Source: CAD feature listing. Evaluate the final solid. Frame: model axes, mm. Face numbers are marked on the shaded views. A direction names the side the tool comes from. Give positions to 0.01 mm unless a question says otherwise; leave off trailing zeros. Order: outer loops, then holes, each group sorted by start corner. A loop starts at its lowest first (then second) coordinate and runs counter-clockwise, first axis right, second up.
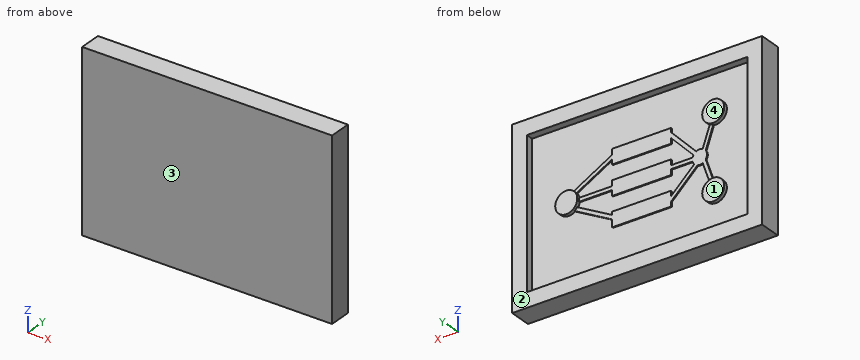
from build123d import *

# Parameters (mm, degrees)
CROQUIS1_W              = 34
CROQUIS1_H              = 24
SALIENTE_EXTRUIR1_DEPTH = 3
CAVIDAD1_START          = 2
CAVIDAD1_OUTLINE_W      = 30
CAVIDAD1_OUTLINE_H      = 20
CAVIDAD1_DEPTH          = 1
CAVIDAD1_START_2        = 2.15
CAVIDAD1_2_DEPTH        = 0.85
CAVIDAD1_START_3        = 2.5
CAVIDAD1_3_OUTLINE_R    = 1.5
CAVIDAD1_3_DEPTH        = 0.5
SALIENTE_EXTRUIR3_DEPTH = 0.5
CROQUIS6_W              = 7.77529117
CROQUIS6_H              = 2
CROQUIS6_W_2            = 2
CROQUIS6_H_2            = 19.575879517
CROQUIS6_W_3            = 7.699177506
CROQUIS6_H_3            = 2.365035227
CROQUIS6_W_4            = 2.895421418
CROQUIS6_W_5            = 7.822528086
CROQUIS6_H_4            = 2.895421418
CROQUIS6_W_6            = 2.695737182
CORTAR_EXTRUIR1_DEPTH   = 0.5


# Read off the part's stored shape, not the designer's step: Cavidad1
with BuildPart() as part:
    # Croquis1 → Saliente-Extruir1 (new body)
    with BuildSketch(Plane(origin=(0, 0, 0), x_dir=(1, 0, 0), z_dir=(0, 1, 0))):
        Rectangle(CROQUIS1_W, CROQUIS1_H)
    extrude(amount=SALIENTE_EXTRUIR1_DEPTH)

    # Cavidad1 outline → Cavidad1 (cut)
    # profile 1 of 3: a face of its own
    with BuildSketch(Plane(origin=(0, 0, 0), x_dir=(1, 0, 0), z_dir=(0, 1, 0)).offset(CAVIDAD1_START)):
        Rectangle(CAVIDAD1_OUTLINE_W, CAVIDAD1_OUTLINE_H)
        with BuildLine():
            Line((-9.751477048, -3.520731146), (-8.727521258, -0.568876422))
            ThreePointArc((-8.727521258, -0.568876422), (-8.905098242, 0), (-8.727521258, 0.568876422))
            Line((-8.727521258, 0.568876422), (-9.751477048, 3.520731146))
            ThreePointArc((-9.751477048, 3.520731146), (-10.491591745, 6.417158268), (-9.279090958, 3.684595061))
            Line((-9.279090958, 3.684595061), (-8.317043268, 0.911208701))
            ThreePointArc((-8.317043268, 0.911208701), (-8.115800994, 0.977550178), (-7.905098242, 1))
            ThreePointArc((-7.905098242, 1), (-7.74739704, 0.987486876), (-7.593642508, 0.950260662))
            Line((-7.593642508, 0.950260662), (-4, 4.391446273))
            Line((-4, 4.391446273), (-4, 5))
            Line((-4, 5), (4, 5))
            Line((4, 5), (4, 3.993093842))
            Line((4, 3.993093842), (9.128751089, 1.221034535))
            ThreePointArc((9.128751089, 1.221034535), (11.497837988, 0.08050691), (9.264650579, -1.307387176))
            Line((9.264650579, -1.307387176), (4, -4.242890617))
            Line((4, -4.242890617), (4, -5))
            Line((4, -5), (-4, -5))
            Line((-4, -5), (-4, -4.453815845))
            Line((-4, -4.453815845), (-7.424912859, -0.87716703))
            ThreePointArc((-7.424912859, -0.87716703), (-7.866968261, -0.999272788), (-8.317043268, -0.911208701))
            Line((-8.317043268, -0.911208701), (-9.279090958, -3.684595061))
            ThreePointArc((-9.279090958, -3.684595061), (-10.491591745, -6.417158268), (-9.751477048, -3.520731146))
        make_face(mode=Mode.SUBTRACT)
    # profile 2 of 3: a face of its own
    with BuildSketch(Plane(origin=(0, 0, 0), x_dir=(1, 0, 0), z_dir=(0, 1, 0)).offset(CAVIDAD1_START)):
        with BuildLine():
            ThreePointArc((8.520980054, 0.25), (8.609737932, 0.563179707), (8.763967569, 0.849837532))
            Line((8.763967569, 0.849837532), (4, 3.424733527))
            Line((4, 3.424733527), (4, 3))
            Line((4, 3), (-4, 3))
            Line((-4, 3), (-4, 3.699176151))
            Line((-4, 3.699176151), (-7.163035026, 0.670329906))
            ThreePointArc((-7.163035026, 0.670329906), (-7.024496987, 0.473858025), (-6.936852406, 0.25))
            Line((-6.936852406, 0.25), (-4, 0.25))
            Line((-4, 0.25), (-4, 1))
            Line((-4, 1), (4, 1))
            Line((4, 1), (4, 0.25))
            Line((4, 0.25), (8.520980054, 0.25))
        make_face()
    # profile 3 of 3: a face of its own
    with BuildSketch(Plane(origin=(0, 0, 0), x_dir=(1, 0, 0), z_dir=(0, 1, 0)).offset(CAVIDAD1_START)):
        with BuildLine():
            Line((4, -3.670417072), (8.851743131, -0.96514567))
            ThreePointArc((8.851743131, -0.96514567), (8.63856539, -0.629679127), (8.520980054, -0.25))
            Line((8.520980054, -0.25), (4, -0.25))
            Line((4, -0.25), (4, -1))
            Line((4, -1), (-4, -1))
            Line((-4, -1), (-4, -0.25))
            Line((-4, -0.25), (-6.936852406, -0.25))
            ThreePointArc((-6.936852406, -0.25), (-6.987424899, -0.397335669), (-7.060265081, -0.535029839))
            Line((-7.060265081, -0.535029839), (-4, -3.730875667))
            Line((-4, -3.730875667), (-4, -3))
            Line((-4, -3), (4, -3))
            Line((4, -3), (4, -3.670417072))
        make_face()
    extrude(amount=CAVIDAD1_DEPTH, mode=Mode.SUBTRACT)

    # Cavidad1 2 outline → Cavidad1 2 (cut)
    with BuildSketch(Plane(origin=(0, 0, 0), x_dir=(1, 0, 0), z_dir=(0, 1, 0)).offset(CAVIDAD1_START_2)):
        with BuildLine():
            ThreePointArc((-8.727521258, 0.568876422), (-8.905098242, 0), (-8.727521258, -0.568876422))
            Line((-8.727521258, -0.568876422), (-9.751477048, -3.520731146))
            ThreePointArc((-9.751477048, -3.520731146), (-9.508408255, -3.582841732), (-9.279090958, -3.684595061))
            Line((-9.279090958, -3.684595061), (-8.317043268, -0.911208701))
            ThreePointArc((-8.317043268, -0.911208701), (-7.866968261, -0.999272788), (-7.424912859, -0.87716703))
            Line((-7.424912859, -0.87716703), (-4, -4.453815845))
            Line((-4, -4.453815845), (-4, -5))
            Line((-4, -5), (4, -5))
            Line((4, -5), (4, -4.242890617))
            Line((4, -4.242890617), (9.264650579, -1.307387176))
            ThreePointArc((9.264650579, -1.307387176), (9.042777207, -1.154869917), (8.851743131, -0.96514567))
            Line((8.851743131, -0.96514567), (4, -3.670417072))
            Line((4, -3.670417072), (4, -3))
            Line((4, -3), (-4, -3))
            Line((-4, -3), (-4, -3.730875667))
            Line((-4, -3.730875667), (-7.060265081, -0.535029839))
            ThreePointArc((-7.060265081, -0.535029839), (-6.987424899, -0.397335669), (-6.936852406, -0.25))
            Line((-6.936852406, -0.25), (-4, -0.25))
            Line((-4, -0.25), (-4, -1))
            Line((-4, -1), (4, -1))
            Line((4, -1), (4, -0.25))
            Line((4, -0.25), (8.520980054, -0.25))
            ThreePointArc((8.520980054, -0.25), (8.5, 0), (8.520980054, 0.25))
            Line((8.520980054, 0.25), (4, 0.25))
            Line((4, 0.25), (4, 1))
            Line((4, 1), (-4, 1))
            Line((-4, 1), (-4, 0.25))
            Line((-4, 0.25), (-6.936852406, 0.25))
            ThreePointArc((-6.936852406, 0.25), (-7.024496987, 0.473858025), (-7.163035026, 0.670329906))
            Line((-7.163035026, 0.670329906), (-4, 3.699176151))
            Line((-4, 3.699176151), (-4, 3))
            Line((-4, 3), (4, 3))
            Line((4, 3), (4, 3.424733527))
            Line((4, 3.424733527), (8.763967569, 0.849837532))
            ThreePointArc((8.763967569, 0.849837532), (8.930137641, 1.051377446), (9.128751089, 1.221034535))
            Line((9.128751089, 1.221034535), (4, 3.993093842))
            Line((4, 3.993093842), (4, 5))
            Line((4, 5), (-4, 5))
            Line((-4, 5), (-4, 4.391446273))
            Line((-4, 4.391446273), (-7.593642508, 0.950260662))
            ThreePointArc((-7.593642508, 0.950260662), (-7.74739704, 0.987486876), (-7.905098242, 1))
            ThreePointArc((-7.905098242, 1), (-8.115800994, 0.977550178), (-8.317043268, 0.911208701))
            Line((-8.317043268, 0.911208701), (-9.279090958, 3.684595061))
            ThreePointArc((-9.279090958, 3.684595061), (-9.508408255, 3.582841732), (-9.751477048, 3.520731146))
            Line((-9.751477048, 3.520731146), (-8.727521258, 0.568876422))
        make_face()
    extrude(amount=CAVIDAD1_2_DEPTH, mode=Mode.SUBTRACT)

    # Cavidad1 3 outline → Cavidad1 3 (cut)
    with BuildSketch(Plane(origin=(0, 0, 0), x_dir=(1, 0, 0), z_dir=(0, 1, 0)).offset(CAVIDAD1_START_3)):
        with Locations((-10, -5)):
            Circle(CAVIDAD1_3_OUTLINE_R)
        with Locations((-10, 5)):
            Circle(CAVIDAD1_3_OUTLINE_R)
        with Locations((10, 0)):
            Circle(CAVIDAD1_3_OUTLINE_R)
    extrude(amount=CAVIDAD1_3_DEPTH, mode=Mode.SUBTRACT)

    # Croquis5 → Saliente-Extruir3 (add)
    with BuildSketch(Plane(origin=(0, 3, 0), x_dir=(1, 0, 0), z_dir=(0, 1, 0))):
        Polygon((-17, 12), (-7, 12), (-7, 10), (-15, 10), (-15, -10), (-7, -10), (-7, -12), (-17, -12), align=None)
        Polygon((7, 12), (17, 12), (17, -12), (7, -12), (7, -10), (15, -10), (15, 10), (7, 10), align=None)
    extrude(amount=SALIENTE_EXTRUIR3_DEPTH)

    # Croquis6 → Cortar-Extruir1 (cut)
    with BuildSketch(Plane(origin=(0, 3.5, 0), x_dir=(1, 0, 0), z_dir=(0, 1, 0))):
        with Locations((-10.887645585, -11)):
            Rectangle(CROQUIS6_W, CROQUIS6_H)
        with Locations((-16, -0.159576746)):
            Rectangle(CROQUIS6_W_2, CROQUIS6_H_2)
        with Locations((-10.887645585, 11)):
            Rectangle(CROQUIS6_W, CROQUIS6_H)
        Polygon((-17, 12), (-17, 9.628363012), (-15, 9.628363012), (-15, 10), (-14.77529117, 10), (-14.77529117, 12), align=None)
        Polygon((-15, -9.947516505), (-17, -9.947516505), (-17, -12), (-14.77529117, -12), (-14.77529117, -10), (-15, -10), align=None)
        with Locations((10.830941942, -11.045685777)):
            Rectangle(CROQUIS6_W_3, CROQUIS6_H_3)
        with Locations((16.128241404, -11.045685777)):
            Rectangle(CROQUIS6_W_4, CROQUIS6_H_3)
        Polygon((17.575952113, -12.22820339), (14.680530695, -12.22820339), (14.680530695, -12.891712404), (17.84219776, -12.891712404), (17.84219776, 13.499887418), (14.680530695, 13.499887418), (14.680530695, 12.667869769), (17.376267877, 12.667869769), (17.376267877, 9.772448351), (14.680530695, 9.772448351), (14.680530695, -9.863168163), (17.575952113, -9.863168163), align=None)
        with Locations((10.769266652, 11.22015906)):
            Rectangle(CROQUIS6_W_5, CROQUIS6_H_4)
        with Locations((16.028399286, 11.22015906)):
            Rectangle(CROQUIS6_W_6, CROQUIS6_H_4)
    extrude(amount=-CORTAR_EXTRUIR1_DEPTH, mode=Mode.SUBTRACT)


solid = part.part
(1) Pin query (flat end, axial travel): pin 1 Ø6 at (x, z) = (3, -2.5) entering from +Y. Return the tip coordinate at first contact, or that it passes through.
(2) Section A-A, the plane x = -1. Return loops of the section in (y, z).
(3) Access query for the marked faces 1 and 2. Directions: +Z, -Z, +X, -X, +Y, -Y. A direction counts if a zero-diameter tool reaches every point of the face in a straight line with its end or side. Return the directions, or none.
(4) Section B-B, the plane z = 7.5. Return loops of the section in (x, y).
(5) Draft query along Z for the marked faces 3 and 4. Return one class per face: +Z half, -Z half, draft (parallel to the pull), parting line (faces both ways), or undercut.
(6) Section D-D, the plane z = -5.5. Return loops of the section in (x, y), plus the area to 3 significant figures.
(7) Line query: line 1 along X through (y, z) = (2.5, -9.75); line 2 along Y through (x, z) = (8.5, 2.25); line 3 along Z through (x, y) = (8, 2.1). Output: solid intervals per line, ascending.
(8) Section C-C, the plane x = 13.5. Return loops of the section in (y, z).
Checks:
1. pin 1: stops at y = 2.15
2. outline: (0, -12) - (3, -12) - (3, -10) - (2, -10) - (2, -5) - (2.15, -5) - (2.15, -3) - (2, -3) - (2, -1) - (2.15, -1) - (2.15, 1) - (2, 1) - (2, 3) - (2.15, 3) - (2.15, 5) - (2, 5) - (2, 10) - (3, 10) - (3, 12) - (0, 12) - close
3. face 1: +Y
3. face 2: +Z, -Z, +X, -X, +Y
4. outline: (-17, 0) - (17, 0) - (17, 3) - (15, 3) - (15, 2) - (-15, 2) - (-15, 3) - (-17, 3) - close
5. face 3: draft
5. face 4: undercut
6. outline: (-17, 0) - (17, 0) - (17, 3) - (15, 3) - (15, 2) - (-8.59, 2) - (-8.59, 2.5) - (-11.41, 2.5) - (-11.41, 2) - (-15, 2) - (-15, 3) - (-17, 3) - close
6. area: 73.4 mm2
7. line 1: x = -17 to -15, 15 to 17
7. line 2: y = 0 to 2
7. line 3: z = -12 to -10, -1.83 to -1.26, -0.25 to 0.25, 1.44 to 2.01, 10 to 12
8. outline: (0, -12) - (3, -12) - (3, -10) - (2, -10) - (2, 10) - (3, 10) - (3, 12) - (0, 12) - close
